from build123d import *

# Parameters (mm, degrees)
BOSS_EXTRUDE1_DEPTH                 = 6.35
F_3_32_0_09375_DIAMETER_HOLE1_D     = 2.38125
F_3_32_0_09375_DIAMETER_HOLE1_DEPTH = 8
F_3_32_0_09375_DIAMETER_HOLE1_TIP   = 0.715399675


with BuildPart() as part:
    # Sketch8 → Boss-Extrude1 (new body)
    with BuildSketch(Plane(origin=(0, 0, 0), x_dir=(0, 0, -1), z_dir=(1, 0, 0))):
        Polygon((-84.484414223, -6.159266037), (-84.484414223, -11.187214329), (98.786832766, 8.217533909), (135.378560096, 8.21091712), (135.196228698, 13.21091712), (98.450522899, 13.209873734), align=None)
    extrude(amount=BOSS_EXTRUDE1_DEPTH)

    # 3/32 (0.09375) Diameter Hole1
    with Locations(Plane(origin=(6.35, 0, 0), x_dir=(0, 0, -1), z_dir=(1, 0, 0))):
        with Locations((-68.484414223, -6.979161178), (30.889527611, 3.542545606), (119.276776099, 10.71046509)):
            Hole(F_3_32_0_09375_DIAMETER_HOLE1_D / 2, depth=F_3_32_0_09375_DIAMETER_HOLE1_DEPTH)
            with Locations((0, 0, -(F_3_32_0_09375_DIAMETER_HOLE1_DEPTH + F_3_32_0_09375_DIAMETER_HOLE1_TIP / 2))):  # 118° drill point
                Cone(0, F_3_32_0_09375_DIAMETER_HOLE1_D / 2, F_3_32_0_09375_DIAMETER_HOLE1_TIP, mode=Mode.SUBTRACT)


solid = part.part
Could you check a few things on this model? Use its own coordinates, in mm. Coordinates: 2 decimals unless noted, no trailing zeros. Order: outer loops, then holes, each group sorted by start corner. A loop starts at its lowest first (then second) coordinate and runs counter-clockwise, first axis right, second up. Notation, with made-up numbers: (16, -35) -> (36, -35) arc R21 ccw to (36, -27) -> close; hole circle Ø11 at (69.5, 1). An arc over 180 degrees is marked (long way). One line per question, with ' | ' between items.
Q1. If I drill on L1, parallel to Y at x = 6.25, z = -115; L2, parallel to Y at x = 3.5, z = 54.5, over which ranges is the centre line in solid material (lowest first)?
Return value:
L1: 8.21 to 13.21 | L2: -8.01 to -2.98
Q2. I'm going to push flat-ended pins straight in: P1, Ø2, axis at x = 3, z = 6, coming from the -Y side; P2, Ø3, axis at x = 5.5, z = -73, coming from the -Y side; P3, Ø2, axis at y = 3.54, z = -30.89, coming from the -X side; P4, Ø3, axis at x = 1.5, z = -95, coming from the -Y side. Where does each tip first touch, or does it pass through?
Return value:
P1: y = -2.98 | P2: y = 5.33 | P3: through | P4: y = 7.66
Q3. Imagine slicing it at B-B on z = 42. Please give me the cut outline in (x, y).
Return value:
outline: (0, -6.69) -> (6.35, -6.69) -> (6.35, -1.66) -> (0, -1.66) -> close
Q4. Imagine slicing it at A-A on x = 3.75. Please give me the cut outline in (y, z).
Return value:
outline: (-11.19, 84.48) -> (8.22, -98.79) -> (8.21, -135.38) -> (13.21, -135.2) -> (13.21, -98.45) -> (-6.16, 84.48) -> close; hole circle Ø2.38 at (-6.98, 68.48); hole circle Ø2.38 at (3.54, -30.89); hole circle Ø2.38 at (10.71, -119.28)
